The model under review builds one solid part; all positions refer to its coordinate system, in mm. Coordinates: 2 decimals unless noted, no trailing zeros. Write each loop counter-clockwise with the first axis right and the second up, starting at its lowest first coordinate (ties: lowest second). Pieces come first, ordered by that corner, then holes. Notation, with made-up numbers: (-33, 60) - (11, 60) arc R31 ccw to (11, 95) - close; hole circle Ø4 at (-28.75, 36). An arc over 180 degrees is marked (long way). Return JSON: item names as keys, results as strings. Group by question number.
(1) For pin 1 Ø1.5 at (x, y) = (0.5, 12) entering from -Z, flat-tipped, find the tip position at first contact; note if it passes through.
(2) We need section A-A on x = 1. State the section outline as (y, z) points, then the cut area to 3 significant figures.
(3) To check wall thickness, follow L1, parallel to Z at x = 0.9, y = 6.5 (3 decimals); L2, parallel to Z at x = -0.35, y = 6.75; L3, parallel to Z at x = -0.4, y = 8. State the ranges of each line that lie inside material, in increasing order. Write a range as from..to.
```python
from build123d import *

# Parameters (mm, degrees)
SKETCH2_R = 1.5


with BuildPart() as part:
    # Sweep1: sweep along a path in Sketch3
    with BuildLine(Plane(origin=(0, 0, 0), x_dir=(0, 0, -1), z_dir=(1, 0, 0))) as sweep1_path:
        Line((-32.4, 12.629185438), (-21.962142643, 6.602885683))
        ThreePointArc((-21.962142643, 6.602885683), (-19.102473217, 6.041490923), (-16.49849985, 7.35))
        ThreePointArc((-16.49849985, 7.35), (-9, 10.5), (-1.50150015, 7.35))
        ThreePointArc((-1.50150015, 7.35), (1.583628924, 6.001835461), (4.74069756, 7.171658805))
        Line((4.74069756, 7.171658805), (16.933371859, 18.266129455))
        ThreePointArc((16.933371859, 18.266129455), (33.792710536, 14.288511628), (24, 0))
        Line((24, 0), (-36, 0))
    # Sketch2 → Sweep1 (sweep)
    with BuildSketch(Plane.XY.offset(36)):
        Circle(SKETCH2_R)
    sweep(path=sweep1_path.line)


solid = part.part
```
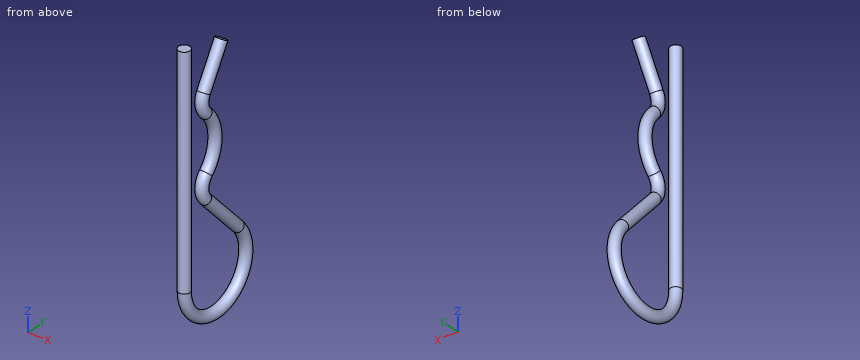
Ans:
{
 "1": {"pin 1": "z = -35.97"},
 "2": {"outline": "(-1.12, -24) arc R11.62 ccw (long way) to (19.09, -16.18) - (8, -3.99) arc R3.38 cw to (8.13, 0.7) arc R11.62 ccw to (8.13, 17.3) arc R3.38 cw to (7.57, 21.4) - (13.6, 31.84) - (11.66, 32.96) - (5.63, 22.52) arc R5.62 ccw to (6.57, 15.7) arc R9.38 cw to (6.57, 2.3) arc R5.62 ccw to (6.34, -5.49) - (17.44, -17.69) arc R9.38 cw (long way) to (1.12, -24) - (1.12, 36) - (-1.12, 36) - close", "area": "355 mm²"},
 "3": {"L1": "-34.995..-32.396, -5.786..2.349, 15.651..24.184", "L2": "-35.36..-32.23, -6.44..2.98, 15.02..25.13", "L3": "-35.68..-32.7, -7.8..-3.47, 0.04..4.76, 13.24..17.96, 21.49..27.27"}
}
